Can you work these out from the model? Positions are in its coordinate system, mm. Face numbers are marked on the shaded views. A direction names the side the tool comes from. Round coordinates to 2 decimals unless told otherwise and drop trailing zeros. Order: outer loops, then holes, each group sorted by start corner. A loop starts at its lowest first (then second) coordinate and runs counter-clockwise, first axis right, second up.
Q1. Will these pins go through, and if not, where does the flat tip stop? P1, Ø4, axis at x = -14, z = -2, coming from the +Y side; P2, Ø1.5, axis at x = -7.5, y = 25, coming from the -Z side; P3, Ø2, axis at y = 10, z = -2.5, coming from the -X side.
Q2. If we section it at B-B (y = 18.5): Please give me the cut outline in (x, z), plus the area to 3 significant figures.
Q3. If we section it at A-A (x = 13.85): Please give me the cut outline in (y, z), plus the area to 3 significant figures.
Q4. If I drill on line 1 (Z direction, x = 13.85, y = 20); line 2 (Z direction, x = -5.32, y = 31.25) (3 decimals); line 3 (X direction, y = 11, z = 3), over which ranges is the centre line in solid material (lowest first)?
Q5. For the marked faces 1, 2, 3 and 4, which set-ups out of +Z, -Z, +X, -X, +Y, -Y let a thin tool reach every point of the face, with its end or its side?
Q6. If we section it at C-C (z = -5.5): Please give me the cut outline in (x, y).
Q7. If we section it at D-D (y = 8): Please give me the cut outline in (x, z), plus the area to 3 significant figures.
from build123d import *

# Parameters (mm, degrees)
SKETCH_1_W               = 22.8
SKETCH_1_H               = 12.16
EXTRUDE_1_DEPTH          = 22.44
EXTRUDE_START            = 18
SKETCH_3_W               = 32.3
SKETCH_3_H               = 12.16
EXTRUDE_2_DEPTH          = 2.52
SKETCH_4_R               = 6.08
SKETCH_4_R_2             = 2.9
EXTRUDE_3_DEPTH          = 6
FILLET_1_R               = 1
SKETCH_5_W               = 2.3
SKETCH_5_H               = 1.2
CUT_EXTRUDE_1_DEPTH      = 2.52
SKETCH_6_R               = 2.3
EXTRUDE_4_DEPTH          = 4.39
HOLE_WIZARD_M2_5_1_D     = 2.05
HOLE_WIZARD_M2_5_1_DEPTH = 4.39
HOLE_WIZARD_M2_5_1_TIP   = 0.615882135
SKETCH_10_W              = 3.6
SKETCH_10_H              = 1.3
EXTRUDE_5_DEPTH          = 2


with BuildPart() as part:
    # Sketch 1 → Extrude 1 (new body)
    with BuildSketch(Plane(origin=(0, 0, 0), x_dir=(1, 0, 0), z_dir=(0, 1, 0))):
        Rectangle(SKETCH_1_W, SKETCH_1_H)
    extrude(amount=EXTRUDE_1_DEPTH)

    # Sketch 3 → Extrude 2 (add)
    with BuildSketch(Plane(origin=(0, 0, 0), x_dir=(1, 0, 0), z_dir=(0, 1, 0)).offset(EXTRUDE_START)):
        Rectangle(SKETCH_3_W, SKETCH_3_H)
    extrude(amount=EXTRUDE_2_DEPTH)

    # Sketch 4 → Extrude 3 (add)
    with BuildSketch(Plane(origin=(0, 22.44, 0), x_dir=(1, 0, 0), z_dir=(0, 1, 0))):
        with Locations((-5.32, 0)):
            Circle(SKETCH_4_R)
        with Locations((0.76, 0)):
            Circle(SKETCH_4_R_2)
    extrude(amount=EXTRUDE_3_DEPTH)

    # Fillet 1
    fillet_1_edges = [part.edges().sort_by_distance(p)[0] for p in [
        (0.068388158, 25.44, -2.816322613),
        (0.068388158, 25.44, 2.816322613),
    ]]
    fillet(fillet_1_edges, radius=FILLET_1_R)

    # Sketch 5 → Cut-Extrude 1 (cut)
    with BuildSketch(Plane(origin=(0, 20.52, 0), x_dir=(1, 0, 0), z_dir=(0, 1, 0))):
        with Locations((-17.3, 0)):
            Rectangle(SKETCH_5_W, SKETCH_5_H)
        with BuildLine():
            Line((-14.65, 0.6), (-16.15, 0.6))
            Line((-16.15, 0.6), (-16.15, -0.6))
            Line((-16.15, -0.6), (-14.65, -0.6))
            ThreePointArc((-14.65, -0.6), (-14.85, 0), (-14.65, 0.6))
        make_face()
        with BuildLine():
            ThreePointArc((-12.85, 0), (-13.533772234, 0.948683298), (-14.65, 0.6))
            Line((-14.65, 0.6), (-13.85, 0.6))
            Line((-13.85, 0.6), (-13.85, -0.6))
            Line((-13.85, -0.6), (-14.65, -0.6))
            ThreePointArc((-14.65, -0.6), (-13.533772234, -0.948683298), (-12.85, 0))
        make_face()
        with BuildLine():
            Line((-13.85, 0.6), (-14.65, 0.6))
            ThreePointArc((-14.65, 0.6), (-14.85, 0), (-14.65, -0.6))
            Line((-14.65, -0.6), (-13.85, -0.6))
            Line((-13.85, -0.6), (-13.85, 0.6))
        make_face()
        with BuildLine():
            ThreePointArc((14.65, 0.6), (12.85, 0), (14.65, -0.6))
            Line((14.65, -0.6), (13.85, -0.6))
            Line((13.85, -0.6), (13.85, 0.6))
            Line((13.85, 0.6), (14.65, 0.6))
        make_face()
        with BuildLine():
            Line((13.85, -0.6), (14.65, -0.6))
            ThreePointArc((14.65, -0.6), (14.798683298, -0.316227766), (14.85, 0))
            ThreePointArc((14.85, 0), (14.798683298, 0.316227766), (14.65, 0.6))
            Line((14.65, 0.6), (13.85, 0.6))
            Line((13.85, 0.6), (13.85, -0.6))
        make_face()
        with BuildLine():
            Line((14.65, -0.6), (18.45, -0.6))
            Line((18.45, -0.6), (18.45, 0.6))
            Line((18.45, 0.6), (14.65, 0.6))
            ThreePointArc((14.65, 0.6), (14.798683298, 0.316227766), (14.85, 0))
            ThreePointArc((14.85, 0), (14.798683298, -0.316227766), (14.65, -0.6))
        make_face()
    extrude(amount=-CUT_EXTRUDE_1_DEPTH, mode=Mode.SUBTRACT)

    # Sketch 6 → Extrude 4 (add)
    with BuildSketch(Plane(origin=(0, 28.44, 0), x_dir=(1, 0, 0), z_dir=(0, 1, 0))):
        with Locations((-5.32, 0)):
            Circle(SKETCH_6_R)
    extrude(amount=EXTRUDE_4_DEPTH)

    # Hole Wizard M2.5 _1
    with Locations(Plane(origin=(0, 32.83, 0), x_dir=(1, 0, 0), z_dir=(0, 1, 0))):
        with Locations((-5.32, 0)):
            Hole(HOLE_WIZARD_M2_5_1_D / 2, depth=HOLE_WIZARD_M2_5_1_DEPTH)
            with Locations((0, 0, -(HOLE_WIZARD_M2_5_1_DEPTH + HOLE_WIZARD_M2_5_1_TIP / 2))):  # 118° drill point
                Cone(0, HOLE_WIZARD_M2_5_1_D / 2, HOLE_WIZARD_M2_5_1_TIP, mode=Mode.SUBTRACT)

    # Sketch 10 → Extrude 5 (add)
    with BuildSketch(Plane.ZY.offset(11.4)):
        with Locations((0, 4.93)):
            Rectangle(SKETCH_10_W, SKETCH_10_H)
    extrude(amount=EXTRUDE_5_DEPTH)


solid = part.part
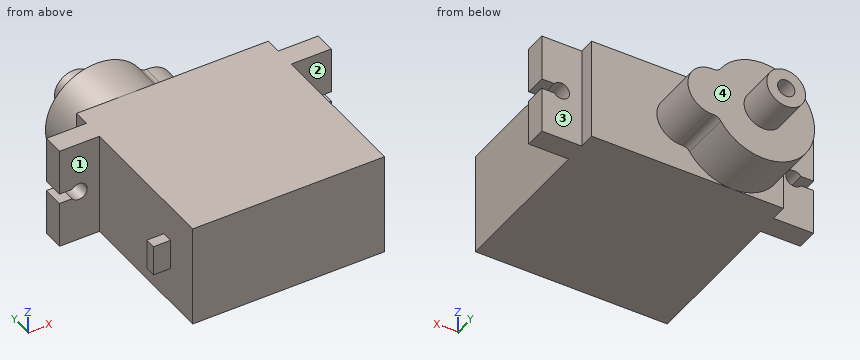
Solution:
1. P1: stops at y = 20.52
1. P2: stops at z = -5.91
1. P3: stops at x = -11.4
2. outline: (-16.15, -6.08) - (16.15, -6.08) - (16.15, -0.6) - (14.65, -0.6) arc R1 cw (long way) to (14.65, 0.6) - (16.15, 0.6) - (16.15, 6.08) - (-16.15, 6.08) - (-16.15, 0.6) - (-14.65, 0.6) arc R1 cw (long way) to (-14.65, -0.6) - (-16.15, -0.6) - close
2. area: 383 mm2
3. outline: (18, -6.08) - (20.52, -6.08) - (20.52, -1) - (18, -1) - close; (18, 1) - (20.52, 1) - (20.52, 6.08) - (18, 6.08) - close
3. area: 25.6 mm2
4. line 1: z = -6.08 to -1, 1 to 6.08
4. line 2: z = -2.3 to -1.025, 1.025 to 2.3
4. line 3: x = -11.4 to 11.4
5. face 1: +Z, -Z, -X
5. face 2: +Z, -Z, +X, -Y
5. face 3: +Z, -Z, +X, +Y
5. face 4: +Y
6. outline: (-16.15, 18) - (-11.4, 18) - (-11.4, 0) - (11.4, 0) - (11.4, 18) - (16.15, 18) - (16.15, 20.52) - (11.4, 20.52) - (11.4, 22.44) - (-2.73, 22.44) - (-2.73, 28.44) - (-7.91, 28.44) - (-7.91, 22.44) - (-11.4, 22.44) - (-11.4, 20.52) - (-16.15, 20.52) - close
7. outline: (-11.4, -6.08) - (11.4, -6.08) - (11.4, 6.08) - (-11.4, 6.08) - close
7. area: 277 mm2
